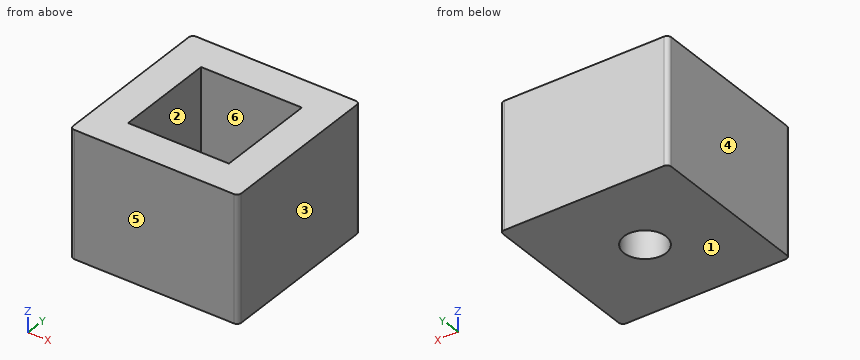
from build123d import *

# Parameters (mm, degrees)
F0_W     = 50.8
F0_H     = 50.8
F0_R     = 6.35
F1_DEPTH = 12.7
F2_W     = 50.8
F2_H     = 50.8
F2_W_2   = 30.48
F2_H_2   = 30.48
F3_DEPTH = 25.4
F4_R     = 1.27


with BuildPart() as f1:
    # F0 (on Top) → F1 (new body)
    with BuildSketch(Plane.XY):
        Rectangle(F0_W, F0_H)
        Circle(F0_R, mode=Mode.SUBTRACT)
    extrude(amount=F1_DEPTH)

    # F2 (on face) → F3 (join)
    with BuildSketch(Plane.XY.offset(12.7)):
        Rectangle(F2_W, F2_H)
        Rectangle(F2_W_2, F2_H_2, mode=Mode.SUBTRACT)
    extrude(amount=F3_DEPTH)

    # F4
    f4_edges = [f1.edges().sort_by_distance(p)[0] for p in [
        (25.4, -25.4, 19.05),
        (25.4, 25.4, 19.05),
        (-25.4, -25.4, 19.05),
        (-25.4, 25.4, 19.05),
    ]]
    fillet(f4_edges, radius=F4_R)


solid = f1.part
Check sheet for the modelled part. Datum: model origin and axes. Units: mm. Face numbers are marked on the shaded views. A direction names the side the tool comes from. Give positions to 0.01 mm unless a question says otherwise; leave off trailing zeros. Write each loop counter-clockwise with the first axis right and the second up, starting at its lowest first coordinate (ties: lowest second). Pieces come first, ordered by that corner, then holes. Notation, with made-up numbers: (41.25, 39.25) -> (50.25, 39.25) arc R24 ccw to (50.25, 52.25) -> close; hole circle Ø7 at (49.5, 45). An arc over 180 degrees is marked (long way). Write item = value, one per line.
Item 1: Tool access check on the marked faces 5 and 6. Record the directions out of +Z, -Z, +X, -X, +Y, -Y that give a thin tool (end or side, any length) a straight path to the whole face; none if there is none.
Output:
face_5 = +Z, -Z, +X, -X, -Y
face_6 = +Z
Item 2: Sectioned sample at D-D on x = -13.5. Record the boundary of the cut face in (y, z), and give its area (3 significant figures).
Output:
outline = (-25.4, 0) -> (25.4, 0) -> (25.4, 38.1) -> (15.24, 38.1) -> (15.24, 12.7) -> (-15.24, 12.7) -> (-15.24, 38.1) -> (-25.4, 38.1) -> close
area = 1,160 mm^2
Item 3: Sectioned sample at B-B on z = 32. Record the boundary of the cut face in (x, y), and give its area (3 significant figures).
Output:
outline = (-25.4, -24.13) arc R1.27 ccw to (-24.13, -25.4) -> (24.13, -25.4) arc R1.27 ccw to (25.4, -24.13) -> (25.4, 24.13) arc R1.27 ccw to (24.13, 25.4) -> (-24.13, 25.4) arc R1.27 ccw to (-25.4, 24.13) -> close; hole (-15.24, -15.24) -> (15.24, -15.24) -> (15.24, 15.24) -> (-15.24, 15.24) -> close
area = 1,650 mm^2
Item 4: Release check for a two-part mould opening along X. For the marked faces 1, 2, 3 and 4 record: +X half, -X half, draft (parallel to the pull), parting line (faces both ways), or undercut.
Output:
face_1 = draft
face_2 = undercut
face_3 = +X half
face_4 = -X half
Item 5: Gauge pin test, flat ends, axial feed: pin 1 (2 mm diameter, centred on x = -12, y = 10.5, fed in from +Z); pin 2 (16.5 mm diameter, centred on x = 0, y = 0, fed in from -Z). Record the tip position at first contact, or that the pin passes through.
Output:
pin_1 = 12.7
pin_2 = 0
Item 6: Scan lines: probe 1 along Y at (x, z) = (0, 8); probe 2 along Y at (x, z) = (-11, 23). Record each from-to range of solid material in increasing order. Write a range as from..to.
Output:
probe_1 = -25.4..-6.35, 6.35..25.4
probe_2 = -25.4..-15.24, 15.24..25.4
Item 7: Sectioned sample at A-A on x = 0. Record the boundary of the cut face in (y, z).
Output:
outline = (-25.4, 0) -> (-6.35, 0) -> (-6.35, 12.7) -> (-15.24, 12.7) -> (-15.24, 38.1) -> (-25.4, 38.1) -> close; (6.35, 0) -> (25.4, 0) -> (25.4, 38.1) -> (15.24, 38.1) -> (15.24, 12.7) -> (6.35, 12.7) -> close
